Build history of the part. All positions in model axes, mm. Face numbers are marked on the shaded views. A direction names the side the tool comes from. Round coordinates to 2 decimals unless told otherwise and drop trailing zeros. Order: outer loops, then holes, each group sorted by start corner. A loop starts at its lowest first (then second) coordinate and runs counter-clockwise, first axis right, second up. Notation, with made-up numbers: (-7, 40) -> (12, 40) arc R7 ccw to (12, 52) -> close; hole circle Ø7 at (17.25, 8.25). An arc over 180 degrees is marked (long way). Write item = value, one per line.
from build123d import *

# Parameters (mm, degrees)
ESQUISSE1_W             = 80
ESQUISSE1_H             = 40
BOSS_EXTRU_1_DEPTH      = 50
ENL_V_MAT_EXTRU_1_DEPTH = 78
ESQUISSE3_W             = 2
ESQUISSE3_H             = 50
BOSS_EXTRU_2_DEPTH      = 40
ESQUISSE4_R             = 11
ENL_V_MAT_EXTRU_2_DEPTH = 81
ESQUISSE5_W             = 60
ESQUISSE5_H             = 36
ENL_V_MAT_EXTRU_3_DEPTH = 48
ESQUISSE6_W             = 10
ESQUISSE6_H             = 5
ENL_V_MAT_EXTRU_4_DEPTH = 2
ENL_V_MAT_EXTRU_5_DEPTH = 10
ESQUISSE8_W             = 10
ESQUISSE8_H             = 9
BOSS_EXTRU_3_DEPTH      = 50
ESQUISSE9_R             = 2.1
ENL_V_MAT_EXTRU_6_DEPTH = 51
ESQUISSE10_R            = 2.1
ENL_V_MAT_EXTRU_7_DEPTH = 20
CONG_1_R                = 4.2
ESQUISSE11_W            = 2
ESQUISSE11_H            = 5
ESQUISSE11_W_2          = 7
ESQUISSE11_H_2          = 2
BOSS_EXTRU_4_DEPTH      = 5


with BuildPart() as part:
    # Esquisse1 → Boss.-Extru.1 (new body)
    with BuildSketch(Plane(origin=(0, 0, 0), x_dir=(1, 0, 0), z_dir=(0, 1, 0))):
        with Locations((40, 20)):
            Rectangle(ESQUISSE1_W, ESQUISSE1_H)
    extrude(amount=BOSS_EXTRU_1_DEPTH)

    # Esquisse2 → Enlèv. mat.-Extru.1 (cut)
    with BuildSketch(Plane.ZY):
        with BuildLine():
            Line((-2, 48), (-38, 48))
            Line((-38, 48), (-38, 2))
            Line((-38, 2), (-32.845232579, 2))
            ThreePointArc((-32.845232579, 2), (-20, 13), (-7.154767421, 2))
            Line((-7.154767421, 2), (-2, 2))
            Line((-2, 2), (-2, 48))
        make_face()
    extrude(amount=-ENL_V_MAT_EXTRU_1_DEPTH, mode=Mode.SUBTRACT)

    # Esquisse3 → Boss.-Extru.2 (add)
    with BuildSketch(Plane(origin=(0, 0, -40), x_dir=(-1, 0, 0), z_dir=(0, 0, -1))):
        with Locations((-1, 25)):
            Rectangle(ESQUISSE3_W, ESQUISSE3_H)
    extrude(amount=-BOSS_EXTRU_2_DEPTH)

    # Esquisse4 → Enlèv. mat.-Extru.2 (cut, through all)
    with BuildSketch(Plane.ZY):
        with Locations((-20, 0)):
            Circle(ESQUISSE4_R)
    extrude(amount=-ENL_V_MAT_EXTRU_2_DEPTH, mode=Mode.SUBTRACT)

    # Esquisse5 → Enlèv. mat.-Extru.3 (cut)
    with BuildSketch(Plane.XZ):
        with Locations((40, -20)):
            Rectangle(ESQUISSE5_W, ESQUISSE5_H)
    extrude(amount=-ENL_V_MAT_EXTRU_3_DEPTH, mode=Mode.SUBTRACT)

    # Esquisse6 → Enlèv. mat.-Extru.4 (cut)
    with BuildSketch(Plane.ZY):
        with Locations((-20, 40.5)):
            Rectangle(ESQUISSE6_W, ESQUISSE6_H)
    extrude(amount=-ENL_V_MAT_EXTRU_4_DEPTH, mode=Mode.SUBTRACT)

    # Esquisse7 → Enlèv. mat.-Extru.5 (cut)
    with BuildSketch(Plane(origin=(80, 0, 0), x_dir=(0, 0, -1), z_dir=(1, 0, 0))):
        with BuildLine():
            Line((17, 24.803847577), (17, 27.021710026))
            Line((17, 27.021710026), (23, 27.021710026))
            Line((23, 27.021710026), (23, 24.803847577))
            ThreePointArc((23, 24.803847577), (25.196152423, 27), (26, 30))
            ThreePointArc((26, 30), (17, 35.196152423), (17, 24.803847577))
        make_face()
        with BuildLine():
            Line((23, 27.021710026), (17, 27.021710026))
            Line((17, 27.021710026), (17, 24.803847577))
            ThreePointArc((17, 24.803847577), (20, 24), (23, 24.803847577))
            Line((23, 24.803847577), (23, 27.021710026))
        make_face()
        with BuildLine():
            ThreePointArc((23, 24.803847577), (20, 24), (17, 24.803847577))
            Line((17, 24.803847577), (17, 10.583005244))
            ThreePointArc((17, 10.583005244), (20, 11), (23, 10.583005244))
            Line((23, 10.583005244), (23, 24.803847577))
        make_face()
    extrude(amount=-ENL_V_MAT_EXTRU_5_DEPTH, mode=Mode.SUBTRACT)

    # Esquisse8 → Boss.-Extru.3 (add)
    with BuildSketch(Plane(origin=(0, 50, 0), x_dir=(1, 0, 0), z_dir=(0, 1, 0))):
        with Locations((5, 4.5)):
            Rectangle(ESQUISSE8_W, ESQUISSE8_H)
        with Locations((5, 35.5)):
            Rectangle(ESQUISSE8_W, ESQUISSE8_H)
        with Locations((75, 35.5)):
            Rectangle(ESQUISSE8_W, ESQUISSE8_H)
        with Locations((75, 4.5)):
            Rectangle(ESQUISSE8_W, ESQUISSE8_H)
    extrude(amount=-BOSS_EXTRU_3_DEPTH)

    # Esquisse9 → Enlèv. mat.-Extru.6 (cut, through all)
    with BuildSketch(Plane(origin=(0, 50, 0), x_dir=(1, 0, 0), z_dir=(0, 1, 0))):
        with Locations((75.8, 4.2)):
            Circle(ESQUISSE9_R)
        with Locations((4.2, 4.2)):
            Circle(ESQUISSE9_R)
        with Locations((4.2, 35.8)):
            Circle(ESQUISSE9_R)
        with Locations((75.8, 35.8)):
            Circle(ESQUISSE9_R)
    extrude(amount=-ENL_V_MAT_EXTRU_6_DEPTH, mode=Mode.SUBTRACT)

    # Esquisse10 → Enlèv. mat.-Extru.7 (cut)
    with BuildSketch(Plane(origin=(0, 50, 0), x_dir=(1, 0, 0), z_dir=(0, 1, 0))):
        Polygon((5.246004718, 39.703742751), (8.103742751, 36.846004718), (8.103742751, 40), (0, 40), (0, 31.896257249), (3.153995282, 31.896257249), (0.296257249, 34.753995282), (1.342261967, 38.657738033), align=None)
        Polygon((7.057738033, 32.942261967), (8.103742751, 36.846004718), (5.246004718, 39.703742751), (1.342261967, 38.657738033), (0.296257249, 34.753995282), (3.153995282, 31.896257249), align=None)
        with Locations((4.2, 35.8)):
            Circle(ESQUISSE10_R, mode=Mode.SUBTRACT)
        Polygon((0.296257249, 5.246004718), (1.342261967, 1.342261967), (5.246004718, 0.296257249), (8.103742751, 3.153995282), (7.057738033, 7.057738033), (3.153995282, 8.103742751), align=None)
        with Locations((4.2, 4.2)):
            Circle(ESQUISSE10_R, mode=Mode.SUBTRACT)
        Polygon((3.153995282, 8.103742751), (0, 8.103742751), (0, 0), (8.103742751, 0), (8.103742751, 3.153995282), (5.246004718, 0.296257249), (1.342261967, 1.342261967), (0.296257249, 5.246004718), align=None)
        Polygon((80, 0), (80, 8.103742751), (76.846004718, 8.103742751), (79.703742751, 5.246004718), (78.657738033, 1.342261967), (74.753995282, 0.296257249), (71.896257249, 3.153995282), (71.896257249, 0), align=None)
        Polygon((72.942261967, 7.057738033), (71.896257249, 3.153995282), (74.753995282, 0.296257249), (78.657738033, 1.342261967), (79.703742751, 5.246004718), (76.846004718, 8.103742751), align=None)
        with Locations((75.8, 4.2)):
            Circle(ESQUISSE10_R, mode=Mode.SUBTRACT)
        Polygon((80, 40), (71.896257249, 40), (71.896257249, 36.846004718), (74.753995282, 39.703742751), (78.657738033, 38.657738033), (79.703742751, 34.753995282), (76.846004718, 31.896257249), (80, 31.896257249), align=None)
        Polygon((74.753995282, 39.703742751), (71.896257249, 36.846004718), (72.942261967, 32.942261967), (76.846004718, 31.896257249), (79.703742751, 34.753995282), (78.657738033, 38.657738033), align=None)
        with Locations((75.8, 35.8)):
            Circle(ESQUISSE10_R, mode=Mode.SUBTRACT)
    extrude(amount=-ENL_V_MAT_EXTRU_7_DEPTH, mode=Mode.SUBTRACT)

    # Congé1
    cong_1_edges = [part.edges().sort_by_distance(p)[0] for p in [
        (0, 15, -40),
        (0, 15, 0),
        (80, 15, 0),
        (80, 15, -40),
    ]]
    fillet(cong_1_edges, radius=CONG_1_R)

    # Esquisse11 → Boss.-Extru.4 (add)
    with BuildSketch(Plane.XZ.offset(-48)):
        with Locations((46, -13.5)):
            Rectangle(ESQUISSE11_W, ESQUISSE11_H)
        Polygon((40, -11), (45, -11), (47, -11), (47, -9), (40, -9), align=None)
        with Locations((46, -26.5)):
            Rectangle(ESQUISSE11_W, ESQUISSE11_H)
        with Locations((43.5, -30)):
            Rectangle(ESQUISSE11_W_2, ESQUISSE11_H_2)
    extrude(amount=BOSS_EXTRU_4_DEPTH)


solid = part.part
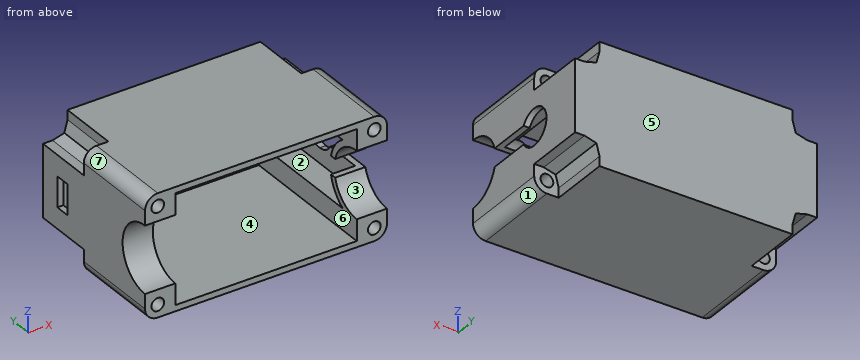
Q1. Cut at C-C, the plane y = 46.5. Give the number of separate pieces and of enclosed holes in the cut face, and give its area (3 significant figures).
Check values:
separate_pieces = 3
enclosed_holes = 1
area = 494 mm²
Q2. Cut at B-B, the plane x = 50.5. List the corners of the cut face in (y, z), and give its area (3 significant figures).
Check values:
outline = (0, -40) -> (50, -40) -> (50, 0) -> (0, 0) -> (0, -2) -> (48, -2) -> (48, -38) -> (0, -38) -> close
area = 272 mm²
Q3. Which spindle directions (+Z, -Z, +X, -X, +Y, -Y) get a long thin tool onto all of the face, cutting with end or side? Do the marked faces 1, 2 and 3. Say none if no direction does.
Check values:
face_1 = -Z, +X, +Y, -Y
face_2 = none
face_3 = +X, -X, -Y
Q4. Flat gauge pins, fed straight in: pin 1 (0.6 mm diameter, centred on x = 1, z = -20, fed in from -Y); pin 2 (1.6 mm diameter, centred on x = 1, y = 40, fed in from +Z); pin 3 (12 mm diameter, centred on x = 21, z = -26.5, fed in from -Y). Where does each tip first touch, or does it go through?
Check values:
pin_1 = 11
pin_2 = -8.1
pin_3 = 48
Q5. Cut at A-A, the plane z = -20. List the corners of the cut face in (x, y), and give its area (3 significant figures).
Check values:
outline = (0, 11) -> (10, 11) -> (10, 13) -> (2, 13) -> (2, 38) -> (0, 38) -> close; (0, 43) -> (2, 43) -> (2, 48) -> (78, 48) -> (78, 36) -> (80, 36) -> (80, 50) -> (0, 50) -> close
area = 264 mm²
Q6. Mould opens along X. For the marked faces 4, 5, 6 and 7 say: released by +X, released by -X, zero draft, split by the parting line, or undercut.
Check values:
face_4 = undercut
face_5 = zero draft
face_6 = undercut
face_7 = released by -X
Q7. Cut at D-D, the plane z = -27. List the corners of the cut face in (x, y).
Check values:
outline = (0, 8.49) -> (10, 8.49) -> (10, 10.95) -> (2, 10.95) -> (2, 48) -> (45, 48) -> (45, 43) -> (47, 43) -> (47, 48) -> (78, 48) -> (78, 10.95) -> (70, 10.95) -> (70, 8.49) -> (80, 8.49) -> (80, 50) -> (0, 50) -> close
Q8. Probe probe 1 along X at (y, z) = (14, -4); probe 2 along Z at (x, y) = (4, 21); probe 3 along Z at (x, y) = (7, 37). List the from-to ranges inside material, lowest first.
Check values:
probe_1 = 0 to 2.11, 6.29 to 10, 70 to 73.71, 77.89 to 80
probe_2 = -40 to -37.89, -33.71 to -31, -9 to -6.29, -2.11 to 0
probe_3 = -32.93 to -31, -9 to -7.07
